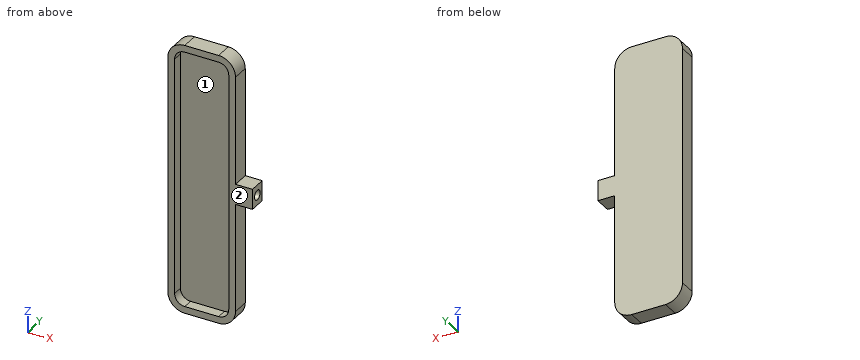
from build123d import *

# Parameters (mm, degrees)
SKETCH1_W           = 20
SKETCH1_H           = 80
BOSS_EXTRUDE1_DEPTH = 5
FILLET1_R           = 5
SHELL1_T            = -2
SKETCH2_W           = 6
SKETCH2_H           = 5
BOSS_EXTRUDE2_DEPTH = 5
SKETCH3_R           = 1.425
CUT_EXTRUDE1_DEPTH  = 4


with BuildPart() as part:
    # Sketch1 → Boss-Extrude1 (new body)
    with BuildSketch(Plane(origin=(0, 0, 0), x_dir=(1, 0, 0), z_dir=(0, 1, 0))):
        Rectangle(SKETCH1_W, SKETCH1_H)
    extrude(amount=BOSS_EXTRUDE1_DEPTH)

    # Fillet1
    fillet1_edges = [part.edges().sort_by_distance(p)[0] for p in [
        (10, 2.5, 40),
        (-10, 2.5, 40),
        (-10, 2.5, -40),
        (10, 2.5, -40),
    ]]
    fillet(fillet1_edges, radius=FILLET1_R)

    # Shell1
    shell1_openings = [part.faces().sort_by_distance(p)[0] for p in [
        (0, 0, 0),
    ]]
    offset(amount=SHELL1_T, openings=shell1_openings, kind=Kind.INTERSECTION)

    # Sketch2 → Boss-Extrude2 (add)
    with BuildSketch(Plane(origin=(10, 0, 0), x_dir=(0, 0, -1), z_dir=(1, 0, 0))):
        with Locations((0, 2.5)):
            Rectangle(SKETCH2_W, SKETCH2_H)
    extrude(amount=BOSS_EXTRUDE2_DEPTH)

    # Sketch3 → Cut-Extrude1 (cut)
    with BuildSketch(Plane(origin=(15, 0, 0), x_dir=(0, 0, -1), z_dir=(1, 0, 0))):
        with Locations((0, 2.5)):
            Circle(SKETCH3_R)
    extrude(amount=-CUT_EXTRUDE1_DEPTH, mode=Mode.SUBTRACT)


solid = part.part
Check sheet for the modelled part. Datum: model origin and axes. Units: mm. Face numbers are marked on the shaded views. A direction names the side the tool comes from. Round coordinates to 2 decimals unless told otherwise and drop trailing zeros. Order: outer loops, then holes, each group sorted by start corner. A loop starts at its lowest first (then second) coordinate and runs counter-clockwise, first axis right, second up.
(1) Access from +Z, -Z, +X, -X, +Y, -Y to the whole of each face (thin tool, end or side, straight path). Record for the marked faces 1 and 2.
(2) Cross-section at A-A, the plane z = 34. Enter the section's corners in (x, y), and give its area (3 significant figures).
(3) Cross-section at C-C, the plane z = 0. Enter the section's corners in (x, y) (3 decimals), and give its area (3 significant figures).
(4) Go/stop test with flat-tipped pins: P1, Ø5, axis at x = -1, z = 19, coming from the -Y side; P2, Ø2.5, axis at x = 12, y = 2.5, coming from the +Z side; P3, Ø1.5, axis at x = -7, y = 2.5, coming from the +Z side. Record where each tip stops, or that it passes through.
(5) Cross-section at B-B, the plane x = 1. Enter the section's corners in (y, z).
(6) Scan lines: probe 1 along X at (y, z) = (2.2, 16); probe 2 along Y at (x, z) = (14.15, 0) (3 decimals); probe 3 along Z at (x, y) = (5.25, 1.6). Record each from-to range of solid material in increasing order.
Check sheet entries:
1. face 1: -Y
1. face 2: +Z, -Z, +X, -X, -Y
2. outline: (-10, 0) - (-8, 0) - (-8, 3) - (8, 3) - (8, 0) - (10, 0) - (10, 5) - (-10, 5) - close
2. area: 52.0 mm2
3. outline: (-10, 0) - (-8, 0) - (-8, 3) - (8, 3) - (8, 0) - (15, 0) - (15, 1.075) - (11, 1.075) - (11, 3.925) - (15, 3.925) - (15, 5) - (-10, 5) - close
3. area: 65.6 mm2
4. P1: stops at y = 3
4. P2: stops at z = 3
4. P3: stops at z = 39.84
5. outline: (0, -40) - (5, -40) - (5, 40) - (0, 40) - (0, 38) - (3, 38) - (3, -38) - (0, -38) - close
6. probe 1: x = -10 to -8, 8 to 10
6. probe 2: y = 0 to 1.075, 3.925 to 5
6. probe 3: z = -39.99 to -37.99, 37.99 to 39.99
